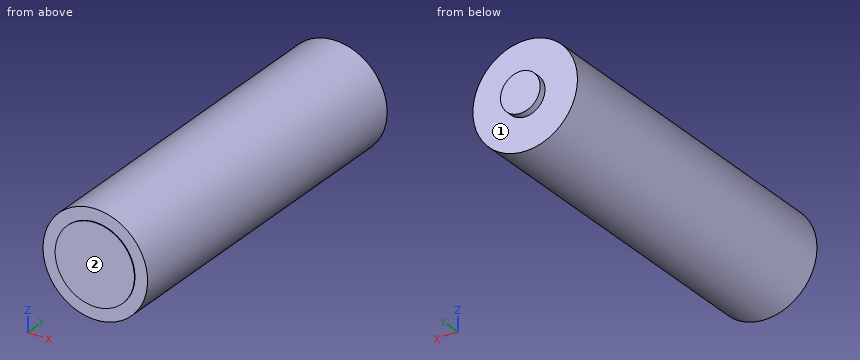
Autodesk Inventor part; units mm, degrees
ref_plane "YZ Plane" through (0, 0, 0) normal (1, 0, 0) x (0, 1, 0)
ref_plane "XZ Plane" through (0, 0, 0) normal (0, 1, 0) x (-1, 0, 0)
ref_plane "XY Plane" through (0, 0, 0) normal (0, 0, 1) x (1, 0, 0)
sketch "Sketch1" plane through (0, 0, 0) normal (0, 1, 0) x (-1, 0, 0)
  circle A0 centre (0, 0) radius 7.25
  dimension "AABatteryDiameter" = 14.5
extrude "Extrusion1" add sketch "Sketch1" along normal blind 49.4
sketch "Sketch2" plane through (0, 49.4, 0) normal (0, 1, 0) x (1, 0, 0)
  circle A0 centre (0, 0) radius 7.25
  circle A1 centre (0, 0) radius 2.75
  dimension "d3" = 5.5
extrude "Extrusion2" add sketch "Sketch2" along normal blind 1 contours A1
sketch "Sketch3" plane through (0, 0, 0) normal (0, -1, 0) x (1, 0, 0)
  circle A0 centre (0, 0) radius 7.25
  circle A1 centre (0, 0) radius 5.5
  dimension "d6" = 11
extrude "Extrusion3" add sketch "Sketch3" along normal blind 0.1 contours A1
equation "\"AABatteryLength\" = d4 + d1 + d7"
properties part number "AABattery"
Read the model definition and answer for the solid it produces. Units are mm, in the model's axes. Face numbers are marked on the shaded views. A direction names the side the tool comes from. Give positions to 0.01 mm unless a question says otherwise; leave off trailing zeros. Order: outer loops, then holes, each group sorted by start corner. A loop starts at its lowest first (then second) coordinate and runs counter-clockwise, first axis right, second up. Notation, with made-up numbers: (64.25, 15) -> (115.25, 15) arc R18 cw to (115.25, 35) -> close; hole circle Ø10 at (-37, 79). An arc over 180 degrees is marked (long way). One line per item, written item: value. Start each with the question number.
(1) The part is cut by section B-B (z = -4.75). Determine the outline of the cut face in (x, y).
(2) The part is cut by section D-D (z = 1.75). Determine the outline of the cut face in (x, y).
(3) A tool of negligible diameter and unlimited length cuts with its end or side. For the marked faces 1 and 2, from which of +Z, -Z, +X, -X, +Y, -Y can it reach the whole face along a straight path? Write none if from no direction.
(4) Flat-ended cylindrical pins translate along their axes: P1, Ø4, axis at y = 21, z = 3.5, coming from the +X side; P2, Ø1.5, axis at y = 22.5, z = -5.5, coming from the +X side; P3, Ø1, axis at y = 17.5, z = 2, coming from the -X side. Find the tip coordinate at first contact, or state that the pin passes through.
(5) Straight lines are drawn through the part: L1, parallel to Y at x = 2.25, z = -3.25; L2, parallel to Y at x = -1, z = -6.25; L3, parallel to Z at x = 2, y = 28. For each, find the intervals that lie inside material, in ascending order.
(6) The part is cut by section C-C (y = 16). Determine the outline of the cut face in (x, z), and give its area (3 significant figures).
(7) The part is cut by section A-A (x = -3.5). Determine the outline of the cut face in (y, z).
Taken from the geometry:
1. outline: (-5.48, 0) -> (-2.77, 0) -> (-2.77, -0.1) -> (2.77, -0.1) -> (2.77, 0) -> (5.48, 0) -> (5.48, 49.4) -> (-5.48, 49.4) -> close
2. outline: (-7.04, 0) -> (-5.21, 0) -> (-5.21, -0.1) -> (5.21, -0.1) -> (5.21, 0) -> (7.04, 0) -> (7.04, 49.4) -> (2.12, 49.4) -> (2.12, 50.4) -> (-2.12, 50.4) -> (-2.12, 49.4) -> (-7.04, 49.4) -> close
3. face 1: +Y
3. face 2: +Z, -Z, +X, -X, -Y
4. P1: x = 7.09
4. P2: x = 5.48
4. P3: x = -7.09
5. L1: -0.1 to 49.4
5. L2: 0 to 49.4
5. L3: -6.97 to 6.97
6. outline: circle Ø14.5 at (0, 0)
6. area: 165 mm^2
7. outline: (-0.1, -4.24) -> (0, -4.24) -> (0, -6.35) -> (49.4, -6.35) -> (49.4, 6.35) -> (0, 6.35) -> (0, 4.24) -> (-0.1, 4.24) -> close
